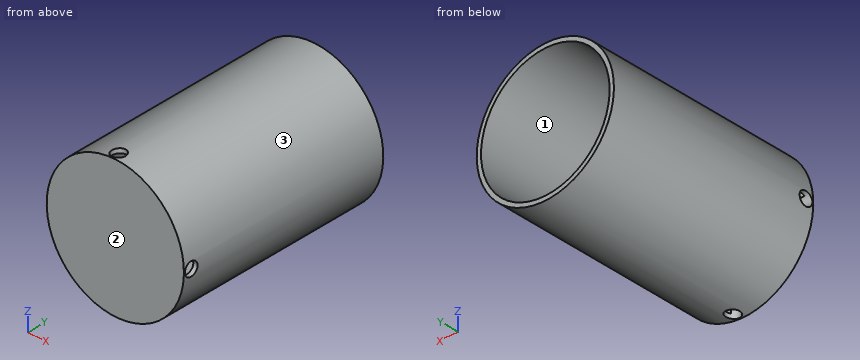
```python
from build123d import *

# Parameters (mm, degrees)
SKETCH1_R                        = 80
BOSS_EXTRUDE1_DEPTH              = 250
SHELL3_T                         = -5
F_16_0MM_DOWEL_HOLE1_D           = 16
F_16_0MM_DOWEL_HOLE1_ON_FACE_2_D = 16


with BuildPart() as part:
    # Sketch1 → Boss-Extrude1 (new body)
    with BuildSketch(Plane(origin=(0, 0, 0), x_dir=(1, 0, 0), z_dir=(0, 1, 0))):
        with Locations(Location((0, 0, 0), (0, 0, 270))):
            Circle(SKETCH1_R)
    extrude(amount=BOSS_EXTRUDE1_DEPTH)

    # Shell3
    shell3_openings = [part.faces().sort_by_distance(p)[0] for p in [
        (0, 250, 0),
    ]]
    offset(amount=SHELL3_T, openings=shell3_openings, kind=Kind.INTERSECTION)

    # Ø16.0mm Dowel Hole1 (through all)
    with Locations(Plane(origin=(79.9948146, 9.136379981, -0.910844193), x_dir=(0.011385552407, 0, 0.999935182498), z_dir=(0.999935182498, 0, -0.011385552407))):
        with Locations((0, 0)):
            Hole(F_16_0MM_DOWEL_HOLE1_D / 2)

    # Ø16.0mm Dowel Hole1 on face 2 (through all)
    with Locations(Plane(origin=(-5.051729974, 9.526351975, 79.840340833), x_dir=(0.998004235716, 0, 0.063147014915), z_dir=(-0.063147014915, 0, 0.998004235716))):
        with Locations((0, 0)):
            Hole(F_16_0MM_DOWEL_HOLE1_ON_FACE_2_D / 2)


solid = part.part
```
Work out the finished part from the listing and answer in its coordinate system (mm). Face numbers are marked on the shaded views. Coordinates: 2 decimals unless noted, no trailing zeros. Loops run counter-clockwise (first coordinate to the right, second up) from the corner with the lowest first, then second, coordinate; pieces in that order, holes last. Notation, with made-up numbers: M 30,-12.75 L 44,-12.75 A36 cw 44,22.25 Z; hole C 79.5,3.5 d5. An arc over 180 degrees is marked long. Use CSV: the item, a comma, the result in double quotes. Start each with the question number.
(1) Find section A-A, the plane y = 150. Give the vertices of the cut face in (x, z), then the cut area to 3 significant figures.
(2) Consider line 1 (Z direction, x = 0, y = 75); line 2 (X direction, y = 153.5, z = 2.5); line 3 (X direction, y = 100.5, z = 63). Determine where each line is inside the solid, lowest interval first.
(3) For a pull along X with two mould halves and no side action, classify the marked faces 1, 2 and 3 as +X half, -X half, draft (parallel to the pull), parting line (faces both ways), or undercut.
(4) Given pin 1 Ø12 at (x, y) = (19, 49.5) entering from +Z; pin 2 Ø8 at (y, z) = (185.5, 59) entering from -X; pin 3 Ø3 at (y, z) = (163.5, 15.5) entering from +X, each flat-ended and moving along its own axis, determine where each tip first touches the part or whether it passes through.
Recorded:
1,outline,"C 0,0 d160; hole C 0,0 d150"
1,area,"2,430 mm^2"
2,line 1,"z = -80 to -75, 75 to 80"
2,line 2,"x = -79.96 to -74.96, 74.96 to 79.96"
2,line 3,"x = -49.31 to -40.69, 40.69 to 49.31"
3,face 1,"undercut"
3,face 2,"draft"
3,face 3,"parting line"
4,pin 1,"stops at z = 78.94"
4,pin 2,"stops at x = -58.09"
4,pin 3,"stops at x = 78.77"
